Read the model definition and answer for the solid it produces. Units are mm, in the model's axes. Face numbers are marked on the shaded views. A direction names the side the tool comes from. Coordinates: 2 decimals unless noted, no trailing zeros. Write each loop counter-clockwise with the first axis right and the second up, starting at its lowest first coordinate (ties: lowest second). Pieces come first, ordered by that corner, then holes. Notation, with made-up numbers: (44, 57) -> (81, 57) arc R17 ccw to (81, 68) -> close; hole circle Ø9 at (-1.75, 30). An arc over 180 degrees is marked (long way). Write item = value, one per line. Start each with the question number.
1) Flat-ended cylindrical pins translate along their axes: pin 1 Ø4 at (y, z) = (17, 6.5) entering from +X; pin 2 Ø9 at (x, y) = (-56, -31) entering from +Z. Find the tip coordinate at first contact, or state that the pin passes through.
2) A tool of negligible diameter and unlimited length cuts with its end or side. For the marked faces 4 and 5, from which of +Z, -Z, +X, -X, +Y, -Y can it reach the whole face along a straight path? Write none if from no direction.
3) Section B-B (z = 23.5) is taken. Determine the outline of the cut face in (x, y), plus the area to 3 significant figures.
4) Section D-D (z = 10) is taken. Determine the outline of the cut face in (x, y).
5) For a pull along Y with two mould halves and no side action, classify the marked faces 1, 2 and 3 as released by +Y, released by -Y, zero draft, split by the parting line, or undercut.
6) Section A-A (x = 22) is taken. Determine the outline of the cut face in (y, z).
7) Find the intervals of material crossed by line 1 along X through (y, z) = (17.5, 13); line 2 along Z through (x, y) = (-50.5, -38.5), in increasing order. Write a range as from..to.
from build123d import *

# Parameters (mm, degrees)
SKETCH1_W           = 80.01
SKETCH1_H           = 80.01
BOSS_EXTRUDE1_DEPTH = 12.827
SKETCH2_R           = 2.032
BOSS_EXTRUDE2_DEPTH = 27.813
SKETCH3_W           = 91.44
SKETCH3_H           = 91.44
SKETCH3_W_2         = 80.01
SKETCH3_H_2         = 80.01
BOSS_EXTRUDE3_DEPTH = 40.64
CUT_EXTRUDE1_DEPTH  = 71.386076528
SKETCH6_W           = 80.518
SKETCH6_H           = 80.518
SKETCH6_W_2         = 80.01
SKETCH6_H_2         = 80.01
CUT_EXTRUDE2_DEPTH  = 27.813
CUT_EXTRUDE3_DEPTH  = 71.386076528
SKETCH9_W           = 19.05
SKETCH9_H           = 19.05
SKETCH9_R           = 3.556
BOSS_EXTRUDE4_DEPTH = 6.35
FILLET1_R           = 9.525
FILLET2_R           = 1.27
FILLET3_R           = 9.525
FILLET4_R           = 1.5875
SKETCH10_R          = 1.27
CUT_EXTRUDE4_DEPTH  = 7.62
CHAMFER2_SIZE       = 6.35


with BuildPart() as part:
    # Sketch1 → Boss-Extrude1 (new body)
    with BuildSketch(Plane.XY):
        Rectangle(SKETCH1_W, SKETCH1_H)
    extrude(amount=BOSS_EXTRUDE1_DEPTH)

    # Sketch2 → Boss-Extrude2 (add)
    with BuildSketch(Plane.XY.offset(12.827)):
        with Locations(Location((-36.068, 36.068, 0), (0, 0, 180))):
            Circle(SKETCH2_R)
        with Locations(Location((36.068, 36.068, 0), (0, 0, 180))):
            Circle(SKETCH2_R)
        with Locations(Location((36.068, -36.068, 0), (0, 0, 180))):
            Circle(SKETCH2_R)
        with Locations(Location((-36.068, -36.068, 0), (0, 0, 180))):
            Circle(SKETCH2_R)
    extrude(amount=BOSS_EXTRUDE2_DEPTH)

    # Sketch3 → Boss-Extrude3 (add, through all)
    with BuildSketch(Plane(origin=(0, 0, 0), x_dir=(-1, 0, 0), z_dir=(0, 0, -1))):
        Rectangle(SKETCH3_W, SKETCH3_H)
        Rectangle(SKETCH3_W_2, SKETCH3_H_2, mode=Mode.SUBTRACT)
    extrude(amount=-BOSS_EXTRUDE3_DEPTH)

    # Sketch4 → Cut-Extrude1 (cut, through all)
    with BuildSketch(Plane.XY.offset(12.827)):
        Polygon((24.13, 40.005), (40.005, 24.13), (40.005, -24.13), (24.13, -40.005), (-24.13, -40.005), (-40.005, -24.13), (-40.005, 24.13), (-24.13, 40.005), align=None)
    extrude(amount=-CUT_EXTRUDE1_DEPTH, mode=Mode.SUBTRACT)

    # Sketch6 → Cut-Extrude2 (cut)
    with BuildSketch(Plane.XY.offset(40.64)):
        Rectangle(SKETCH6_W, SKETCH6_H)
        Rectangle(SKETCH6_W_2, SKETCH6_H_2, mode=Mode.SUBTRACT)
    extrude(amount=-CUT_EXTRUDE2_DEPTH, mode=Mode.SUBTRACT)

    # Sketch7 → Cut-Extrude3 (cut, through all)
    with BuildSketch(Plane.XY.offset(12.827)):
        Polygon((-40.259, 24.235210245), (-40.259, -24.235210245), (-24.235210245, -40.259), (24.235210245, -40.259), (40.259, -24.235210245), (40.259, 24.235210245), (24.235210245, 40.259), (-24.235210245, 40.259), align=None)
        Polygon((-40.005, 24.13), (-40.005, -24.13), (-24.13, -40.005), (24.13, -40.005), (40.005, -24.13), (40.005, 24.13), (24.13, 40.005), (-24.13, 40.005), align=None, mode=Mode.SUBTRACT)
    extrude(amount=-CUT_EXTRUDE3_DEPTH, mode=Mode.SUBTRACT)

    # Sketch9 → Boss-Extrude4 (add)
    # profile 1 of 2: a face of its own
    with BuildSketch(Plane(origin=(0, 0, 0), x_dir=(-1, 0, 0), z_dir=(0, 0, -1))):
        with Locations((55.245, -36.195)):
            Rectangle(SKETCH9_W, SKETCH9_H)
        with Locations((55.245, -36.195)):
            Circle(SKETCH9_R, mode=Mode.SUBTRACT)
    # profile 2 of 2: a face of its own
    with BuildSketch(Plane(origin=(0, 0, 0), x_dir=(-1, 0, 0), z_dir=(0, 0, -1))):
        with Locations((55.245, 36.195)):
            Rectangle(SKETCH9_W, SKETCH9_H)
        with Locations(Location((55.245, 36.195, 0), (0, 0, 180))):
            Circle(SKETCH9_R, mode=Mode.SUBTRACT)
    boss_extrude4 = extrude(amount=-BOSS_EXTRUDE4_DEPTH)

    # Fillet1
    fillet1_edges = [part.edges().sort_by_distance(p)[0] for p in [
        (-45.72, 26.67, 3.175),
        (-45.72, -26.67, 3.175),
        (-64.77, -45.72, 3.175),
        (-64.77, -26.67, 3.175),
        (-64.77, 26.67, 3.175),
        (-64.77, 45.72, 3.175),
    ]]
    fillet(fillet1_edges, radius=FILLET1_R - 0.0001)  # a hair under: the kernel refuses the full size

    # Fillet2
    fillet2_edges = [part.edges().sort_by_distance(p)[0] for p in [
        (-45.72, -31.43255, 6.35),
        (-45.72, 31.43255, 6.35),
    ]]
    fillet(fillet2_edges, radius=FILLET2_R)

    # Mirror4: Boss-Extrude4 across plane
    add(boss_extrude4.mirror(Plane(origin=(0, 0, 0), x_dir=(0, 0, 1), z_dir=(1, 0, 0))))

    # Fillet3
    fillet3_edges = [part.edges().sort_by_distance(p)[0] for p in [
        (45.72, -26.67, 3.175),
        (64.77, -26.67, 3.175),
        (64.77, -45.72, 3.175),
        (45.72, 26.67, 3.175),
        (64.77, 26.67, 3.175),
        (64.77, 45.72, 3.175),
    ]]
    fillet(fillet3_edges, radius=FILLET3_R - 0.0001)  # a hair under: the kernel refuses the full size

    # Fillet4
    fillet4_edges = [part.edges().sort_by_distance(p)[0] for p in [
        (45.72, -31.43255, 6.35),
        (45.72, 31.43255, 6.35),
    ]]
    fillet(fillet4_edges, radius=FILLET4_R)

    # Sketch10 → Cut-Extrude4 (cut)
    with BuildSketch(Plane.XY.offset(40.64)):
        with Locations((-42.545, 42.545)):
            Circle(SKETCH10_R)
        with Locations((42.545, 42.545)):
            Circle(SKETCH10_R)
        with Locations((42.545, -42.545)):
            Circle(SKETCH10_R)
        with Locations((-42.545, -42.545)):
            Circle(SKETCH10_R)
    extrude(amount=-CUT_EXTRUDE4_DEPTH, mode=Mode.SUBTRACT)

    # Chamfer2
    chamfer2_edges = [part.edges().sort_by_distance(p)[0] for p in [
        (-32.247105122, 32.247105122, 0),
        (32.247105122, 32.247105122, 0),
        (32.247105122, -32.247105122, 0),
        (-32.247105122, -32.247105122, 0),
    ]]
    chamfer(chamfer2_edges, length=CHAMFER2_SIZE)


solid = part.part
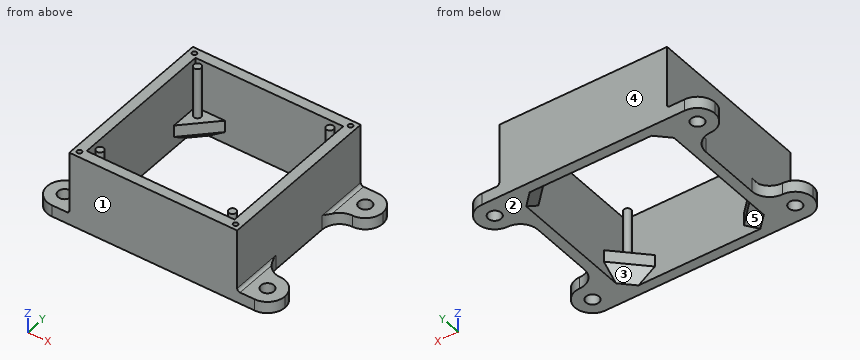
Answer key:
q1.pin_1 = 45.9
q1.pin_2 = 6.35
q2.face_4 = +Z, -Z, +X, -X, +Y
q2.face_5 = -Z
q3.outline = (-45.72, -45.72) -> (45.72, -45.72) -> (45.72, 45.72) -> (-45.72, 45.72) -> close; circle Ø4.06 at (-36.07, -36.07); circle Ø4.06 at (-36.07, 36.07); circle Ø4.06 at (36.07, -36.07); circle Ø4.06 at (36.07, 36.07); hole (-40.26, -40.26) -> (40.26, -40.26) -> (40.26, 40.26) -> (-40.26, 40.26) -> close
q3.area = 1,930 mm^2
q4.outline = (-45.72, -45.72) -> (45.72, -45.72) -> (45.72, 45.72) -> (-45.72, 45.72) -> close; hole (-40.26, -24.24) -> (-24.24, -40.26) -> (24.24, -40.26) -> (40.26, -24.24) -> (40.26, 24.24) -> (24.24, 40.26) -> (-24.24, 40.26) -> (-40.26, 24.24) -> close
q5.face_1 = released by -Y
q5.face_2 = zero draft
q5.face_3 = undercut
q6.outline = (-45.72, 0) -> (-40.26, 0) -> (-40.26, 40.64) -> (-45.72, 40.64) -> close; (40.26, 0) -> (45.72, 0) -> (45.72, 40.64) -> (40.26, 40.64) -> close
q7.line_1 = -45.72..-40.26, 40.26..45.72
q7.line_2 = 0..6.35
